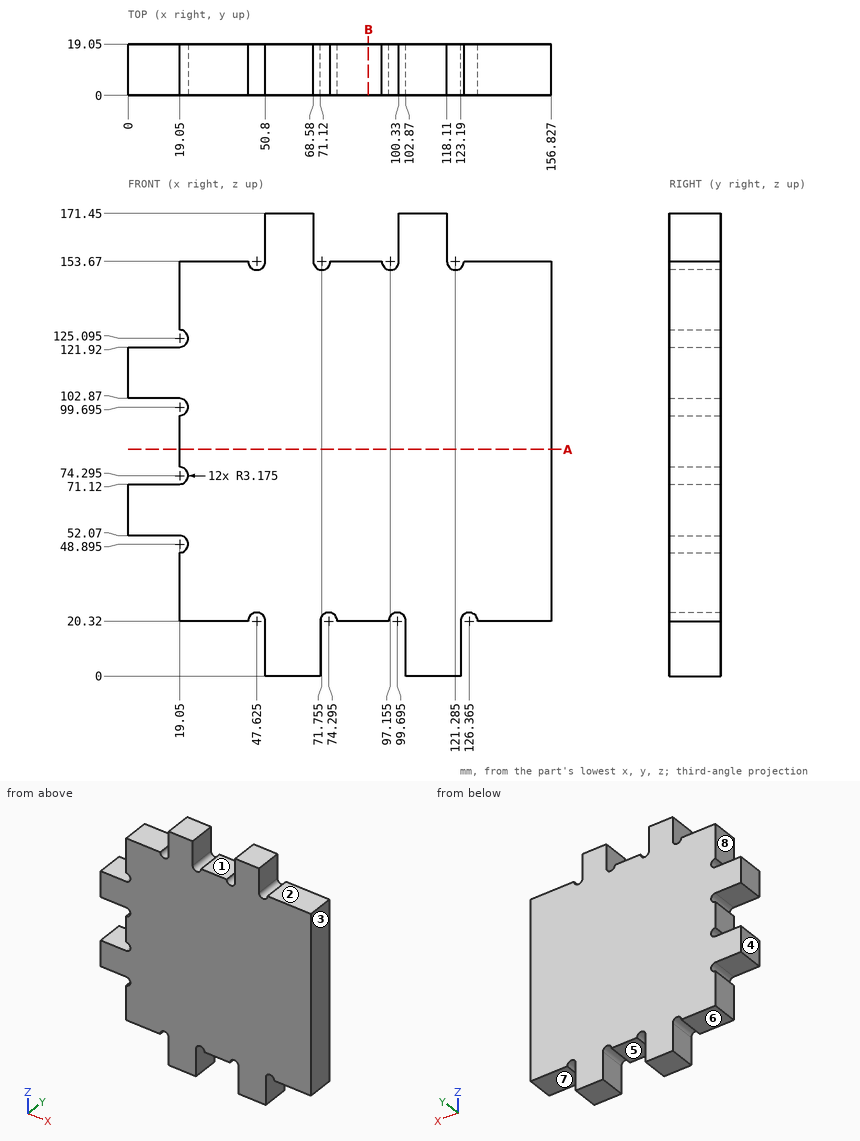
Check sheet for the drawn part. Datum: minimum x, y, z corner. Units: mm. A direction names the side the tool comes from. Round coordinates to 2 decimals unless told otherwise and drop trailing zeros. Order: outer loops, then holes, each group sorted by start corner. A loop starts at its lowest first (then second) coordinate and runs counter-clockwise, first axis right, second up.
(1) Access from +Z, -Z, +X, -X, +Y, -Y to the whole of each face (thin tool, end or side, straight path). Record for the marked faces 5, 6, 7 and 8.
(2) Go/stop test with flat-tipped pins: P1, Ø5.5, axis at y = 13, z = 13.5, coming from the +X side; P2, Ø9.5, axis at x = 12.5, y = 5.5, coming from the +Z side; P3, Ø9.5, axis at y = 5, z = 7.5, coming from the -X side. Record where each tip stops, or that it passes through.
(3) Cross-section at A-A, the plane z = 84. Enter the section's corners in (x, y), and give its area (3 significant figures).
(4) Draft check along X on the marked faces 1, 2, 3 and 4. Enter one of: pulls with the +X half, pulls with the -X half, needs draft (parallel to the pull), parting line crosses it, or undercut.
(5) Cross-section at B-B, the plane x = 89. Enter the section's corners in (y, z).
(6) Scan lines: probe 1 along X at (y, z) = (12, 20); probe 2 along X at (y, z) = (8, 155.5); probe 3 along X at (y, z) = (15.25, 153). Record each from-to range of solid material in increasing order.
Check sheet entries:
1. face 5: -Z, +Y, -Y
1. face 6: -Z, -X, +Y, -Y
1. face 7: -Z, +X, +Y, -Y
1. face 8: +Z, -X, +Y, -Y
2. P1: stops at x = 123.19
2. P2: stops at z = 121.92
2. P3: stops at x = 50.8
3. outline: (19.05, 0) - (156.83, 0) - (156.83, 19.05) - (19.05, 19.05) - close
3. area: 2,620 mm2
4. face 1: undercut
4. face 2: needs draft
4. face 3: pulls with the +X half
4. face 4: pulls with the -X half
5. outline: (0, 20.32) - (19.05, 20.32) - (19.05, 153.67) - (0, 153.67) - close
6. probe 1: x = 50.8 to 71.12, 102.87 to 123.19
6. probe 2: x = 50.8 to 68.58, 100.33 to 118.11
6. probe 3: x = 19.05 to 44.52, 50.73 to 68.65, 74.86 to 94.05, 100.26 to 118.18, 124.39 to 156.83
